from build123d import *

# Parameters (mm, degrees)
F0_W     = 53.655
F0_H     = 28.74146271
F1_W     = 48.9
F1_H     = 28.74146271
F6_D     = 3.8862
F6_DEPTH = 53.656
F7_D     = 3.8862
F7_DEPTH = 53.6560001


with BuildPart() as f4:
    # F0 (on Right) → F4 (revolve)
    with BuildSketch(Plane.YZ):
        with Locations((26.8275, -14.370731355)):
            Rectangle(F0_W, F0_H)
    revolve(axis=Axis((0, 0, -14.370731355), (0, 0, -1)))

    # F1 (on Front) → F5 (revolve, cut)
    with BuildSketch(Plane.XZ):
        with Locations((24.45, -14.370731355)):
            Rectangle(F1_W, F1_H)
    revolve(axis=Axis((0, 0, -14.370731355), (0, 0, -1)), mode=Mode.SUBTRACT)

    # F6 (through all, one way)
    with BuildSketch(Plane(origin=(0, 0, 0), x_dir=(0, 1, 0), z_dir=(-1, 0, 0))):
        with Locations((0, 14.370731355)):
            Circle(F6_D / 2)
    extrude(amount=-F6_DEPTH, mode=Mode.SUBTRACT)

    # F7 (through all, one way)
    with BuildSketch(Plane.XZ):
        with Locations((0, -14.370731355)):
            Circle(F7_D / 2)
    extrude(amount=-F7_DEPTH, mode=Mode.SUBTRACT)


solid = f4.part
Verification items for the finished model (mm, model axes). A direction names the side the tool comes from. Give positions to 0.01 mm unless a question says otherwise; leave off trailing zeros. Loops run counter-clockwise (first coordinate to the right, second up) from the corner with the lowest first, then second, coordinate; pieces in that order, holes last. Notation, with made-up numbers: (-15, 73) - (-4, 73) arc R16 ccw to (-4, 103) - close; hole circle Ø3 at (17, -26.75). An arc over 180 degrees is marked (long way). Write each question's results on one line, items separated by ' | '.
1) Depth check by flat-ended pin: P1, Ø8, axis at x = 1, z = -14, coming from the +Y side (3 decimals); P2, Ø12, axis at y = -19.5, z = -11.5, coming from the -X side; P3, Ø4, axis at x = -31, z = -7.5, coming from the -Y side; P4, Ø10, axis at x = 35.5, z = -26, coming from the +Y side. Enter the tip coordinate at first touch or a pass-through.
Solution:
P1: y = 53.655 | P2: x = -51.93 | P3: y = -45.14 | P4: y = 44.14
2) Sectioned sample at A-A on y = 0. Record the boundary of the cut face in (x, z) (3 decimals), plus the area to 3 significant figures.
Solution:
outline: (-53.655, -28.741) - (-48.9, -28.741) - (-48.9, 0) - (-53.655, 0) - close; (48.9, -28.741) - (53.655, -28.741) - (53.655, -16.314) - (48.9, -16.314) - close; (48.9, -12.428) - (53.655, -12.428) - (53.655, 0) - (48.9, 0) - close | area: 255 mm2
3) Sectioned sample at D-D on x = -32.5. Record the boundary of the cut face in (y, z).
Solution:
outline: (-42.69, -28.74) - (-36.54, -28.74) - (-36.54, 0) - (-42.69, 0) - close; (36.54, -28.74) - (42.69, -28.74) - (42.69, 0) - (36.54, 0) - close
4) Tool access check on faces 1 (the flat face through (-43, -24, 0)), 2 (the cylindrical face through (51.225, -0.421, -12.474)). Record the directions out of +Z, -Z, +X, -X, +Y, -Y that give a thin tool (end or side, any length) a straight path to the whole face; none if there is none.
Solution:
face 1: +Z, +X, -X, +Y, -Y | face 2: +X
5) Material ranges on L1, parallel to X at y = 0.5, z = -12; L2, parallel to Z at x = 51.7, y = 0; L3, parallel to X at y = -1.5, z = -17.5, recorded low to high. Write a range as from..to.
Solution:
L1: -53.65..-48.9, 48.9..53.65 | L2: -28.74..-16.31, -12.43..0 | L3: -53.63..-48.88, 48.88..53.63
6) Mould release check, pull along X, two halves, no side actions. Record for faces 3 (the flat face through (-43, -24, -28.741)), 4 (the cylindrical face through (53.2, -6.98, -14.17)), 5 (the cylindrical face through (-0.253, 51.224, -12.444)): pulls with the +X half, pulls with the -X half, needs draft (parallel to the pull), parting line crosses it, or undercut.
Solution:
face 3: needs draft | face 4: parting line crosses it | face 5: undercut
7) Sectioned sample at C-C on y = -18.5. Record the boundary of the cut face in (x, z), plus the area to 3 significant figures.
Solution:
outline: (-50.36, -28.74) - (-45.27, -28.74) - (-45.27, 0) - (-50.36, 0) - close; (45.27, -28.74) - (50.36, -28.74) - (50.36, 0) - (45.27, 0) - close | area: 293 mm2
